from build123d import *

# Parameters (mm, degrees)
SKETCH1_R           = 27.5
SKETCH1_R_2         = 2.778125
SKETCH1_R_3         = 12.7
BOSS_EXTRUDE1_DEPTH = 7.5
CHAMFER1_SIZE       = 0.5


with BuildPart() as part:
    # Sketch1 → Boss-Extrude1 (new body)
    with BuildSketch(Plane.XY):
        Circle(SKETCH1_R)
        with Locations((-9.5170625, 16.484035789)):
            Circle(SKETCH1_R_2, mode=Mode.SUBTRACT)
        with Locations((19.034125, 0)):
            Circle(SKETCH1_R_2, mode=Mode.SUBTRACT)
        with Locations((-9.5170625, -16.484035789)):
            Circle(SKETCH1_R_2, mode=Mode.SUBTRACT)
        Circle(SKETCH1_R_3, mode=Mode.SUBTRACT)
    extrude(amount=BOSS_EXTRUDE1_DEPTH)

    # Chamfer1
    chamfer1_edges = [part.edges().sort_by_distance(p)[0] for p in [
        (-27.5, 0, 7.5),
    ]]
    chamfer(chamfer1_edges, length=CHAMFER1_SIZE)


solid = part.part
Read the model definition and answer for the solid it produces. Units are mm, in the model's axes. Round coordinates to 2 decimals unless told otherwise and drop trailing zeros. Write each loop counter-clockwise with the first axis right and the second up, starting at its lowest first coordinate (ties: lowest second). Pieces come first, ordered by that corner, then holes. Notation, with made-up numbers: (71, 5.25) - (115, 5.25) arc R28 cw to (115, 44.25) - close; hole circle Ø9 at (41, 6). An arc over 180 degrees is marked (long way). Use a Markdown table: item, result.
(1) The part is cut by section A-A (x = 0). Write down the section's boundary in (y, z), then the cut area to 3 significant figures.
Reported:
| item | result |
|---|---|
| outline | (-27.5, 0) - (-12.7, 0) - (-12.7, 7.5) - (-27, 7.5) - (-27.5, 7) - close; (12.7, 0) - (27.5, 0) - (27.5, 7) - (27, 7.5) - (12.7, 7.5) - close |
| area | 222 mm2 |
(2) The part is cut by section B-B (y = 0). Write down the section's boundary in (x, z).
Reported:
| item | result |
|---|---|
| outline | (-27.5, 0) - (-12.7, 0) - (-12.7, 7.5) - (-27, 7.5) - (-27.5, 7) - close; (12.7, 0) - (16.26, 0) - (16.26, 7.5) - (12.7, 7.5) - close; (21.81, 0) - (27.5, 0) - (27.5, 7) - (27, 7.5) - (21.81, 7.5) - close |
(3) Straight lines are drawn through the part: line 1 along Y through (x, z) = (-9, 2.5); line 2 along Y through (x, z) = (0, 5.25); line 3 along X through (y, z) = (-9.5, 1). For each, find the intervals that lie inside material, in ascending order. Write a range as [from, to].
Reported:
| item | result |
|---|---|
| line 1 | [-25.99, -19.21], [-13.75, -8.96], [8.96, 13.75], [19.21, 25.99] |
| line 2 | [-27.5, -12.7], [12.7, 27.5] |
| line 3 | [-25.81, -8.43], [8.43, 25.81] |
(4) The mould has two halves that part along X. Classify faces 1 (the flat face through (6, -12, 7.5)), 2 (the cylindrical face through (-5.961, -26.846, 3.451)), 3 (the cylindrical face through (-11.72, 14.79, 3.7)): released by +X, released by -X, zero draft, split by the parting line, or undercut.
Reported:
| item | result |
|---|---|
| face 1 | zero draft |
| face 2 | split by the parting line |
| face 3 | undercut |
(5) Each of these flat-tipped pins is pushed along its axis until it touches: pin 1 Ø10 at (x, y) = (14, -20.5) entering from -Z; pin 2 Ø2 at (y, z) = (9, 2) entering from +X; pin 3 Ø4 at (y, z) = (-4.5, 1.5) entering from -X. Where does it stop, or does it pass through?
Reported:
| item | result |
|---|---|
| pin 1 | z = 0 |
| pin 2 | x = 26.31 |
| pin 3 | x = -27.39 |
(6) The part is cut by section D-D (x = -11). State how many separate pieces and enclosed holes the cut face has, then the cut area to 3 significant figures.
Reported:
| item | result |
|---|---|
| separate pieces | 4 |
| enclosed holes | 0 |
| area | 212 mm2 |
(7) The part is cut by section C-C (z = 4.25). Write down the section's boundary in (x, y), then the cut area to 3 significant figures.
Reported:
| item | result |
|---|---|
| outline | circle Ø55 at (0, 0); hole circle Ø25.4 at (0, 0); hole circle Ø5.56 at (-9.52, -16.48); hole circle Ø5.56 at (-9.52, 16.48); hole circle Ø5.56 at (19.03, 0) |
| area | 1,800 mm2 |
